Autodesk Inventor part; units mm, degrees
ref_plane "YZ Plane" through (0, 0, 0) normal (1, 0, 0) x (0, 1, 0)
ref_plane "XZ Plane" through (0, 0, 0) normal (0, 1, 0) x (-1, 0, 0)
ref_plane "XY Plane" through (0, 0, 0) normal (0, 0, 1) x (1, 0, 0)
sketch "Sketch6" plane through (0, 0, 0) normal (0, 1, 0) x (-1, 0, 0)
  line L0 (4.5, -6.1) -> (60.5, -6.1)
  line L1 (60.5, -6.1) -> (60.5, -90.9)
  line L2 (4.5, -90.9) -> (4.5, -6.1)
  line L3 (65.1201, -97) -> (0, -97)
  line L4 (0, -97) -> (0, 0)
  line L5 (0, 0) -> (65.1201, 0)
  line L6 (65.1201, 0) -> (65.1201, -97)
  line L7 (60.5, -90.9) -> (4.5, -90.9)
  line L8 (102.5, -48.5) -> (-37.5, -48.5)
  line L9 (32.5, -118.5) -> (32.5, 21.5)
  circle A0 centre (32.5, -48.5) radius 70
  line L10 (102.5, -48.5) -> (67.5, -109.1218)
  line L11 (67.5, -109.1218) -> (-2.5, -109.1218)
  line L12 (-2.5, -109.1218) -> (-37.5, -48.5)
  line L13 (-37.5, -48.5) -> (-2.5, 12.1218)
  line L14 (-2.5, 12.1218) -> (67.5, 12.1218)
  line L15 (67.5, 12.1218) -> (102.5, -48.5)
  line L16 (32.5, 12.1218) -> (85, -18.1891)
  line L17 (85, -18.1891) -> (85, -78.8109)
  line L18 (85, -78.8109) -> (32.5, -109.1218)
  line L19 (32.5, -109.1218) -> (-20, -78.8109)
  line L20 (-20, -78.8109) -> (-20, -18.1891)
  line L21 (-20, -18.1891) -> (32.5, 12.1218)
  line L22 (32.5, 12.1218) -> (47.5, 12.1218)
  line L23 (47.5, 12.1218) -> (47.5, 5.6218)
  line L24 (47.5, 5.6218) -> (17.5, 5.6218)
  line L25 (17.5, 5.6218) -> (17.5, 12.1218)
  line L26 (47.5, 5.6218) -> (56.6924, 5.6218) construction
  line L27 (17.5, 8.8718) -> (20, 8.8718)
  line L28 (47.5, 8.8718) -> (45, 8.8718)
  line L29 (45, 8.8718) -> (45, 10.1218)
  line L30 (45, 10.1218) -> (20, 10.1218)
  line L31 (20, 10.1218) -> (20, 7.6218)
  line L32 (20, 7.6218) -> (45, 7.6218)
  line L33 (45, 7.6218) -> (45, 10.1218)
  line L34 (67.5, 12.1218) -> (32.5, -48.5)
  line L35 (32.5, -48.5) -> (67.5, -109.1218)
  line L36 (47.5, 5.6218) -> (56.6924, 5.6218)
  line L37 (17.5, 5.6218) -> (11, 5.6218)
  line L38 (17.5, 12.1218) -> (11, 5.6218)
  line L39 (17.5, 12.1218) -> (26.6924, 12.1218) construction
  line L40 (47.5, 12.1218) -> (54, 5.6218)
  line L41 (85, -18.1891) -> (77.5, -5.1987)
  line L42 (77.5, -5.1987) -> (71.8708, -8.4487)
  line L43 (71.8708, -8.4487) -> (86.8708, -34.4295)
  line L44 (86.8708, -34.4295) -> (92.5, -31.1795)
  line L45 (71.8708, -8.4487) -> (67.2746, -0.4879) construction
  line L46 (89.6854, -32.8045) -> (88.4354, -30.6394)
  line L47 (74.6854, -6.8237) -> (75.9354, -8.9888)
  line L48 (75.9354, -8.9888) -> (77.0179, -8.3638)
  line L49 (77.0179, -8.3638) -> (89.5179, -30.0144)
  line L50 (89.5179, -30.0144) -> (87.3529, -31.2644)
  line L51 (87.3529, -31.2644) -> (74.8529, -9.6138)
  line L52 (74.8529, -9.6138) -> (77.0179, -8.3638)
  line L53 (71.8708, -8.4487) -> (67.2746, -0.4879)
  line L54 (86.8708, -34.4295) -> (90.1208, -40.0587)
  line L55 (92.5, -31.1795) -> (90.1208, -40.0587)
  line L56 (92.5, -31.1795) -> (87.9038, -23.2187) construction
  line L57 (77.5, -5.1987) -> (68.6208, -2.8196)
  line L58 (71.8708, -88.5513) -> (67.2746, -96.5121) construction
  line L59 (74.6854, -90.1763) -> (75.9354, -88.0112)
  line L60 (74.8529, -87.3862) -> (77.0179, -88.6362)
  line L61 (77.5, -91.8013) -> (71.8708, -88.5513)
  line L62 (77.5, -91.8013) -> (68.6208, -94.1804)
  line L63 (71.8708, -88.5513) -> (67.2746, -96.5121)
  line L64 (77.0179, -88.6362) -> (89.5179, -66.9856)
  line L65 (87.3529, -65.7356) -> (74.8529, -87.3862)
  line L66 (71.8708, -88.5513) -> (86.8708, -62.5705)
  line L67 (89.5179, -66.9856) -> (87.3529, -65.7356)
  line L68 (89.6854, -64.1955) -> (88.4354, -66.3606)
  line L69 (86.8708, -62.5705) -> (92.5, -65.8205)
  line L70 (86.8708, -62.5705) -> (90.1208, -56.9413)
  line L71 (92.5, -65.8205) -> (90.1208, -56.9413)
  line L72 (94.9944, -48.5) -> (63.7472, -102.6218)
  line L73 (63.7472, -102.6218) -> (1.2528, -102.6218)
  line L74 (1.2528, -102.6218) -> (-29.9944, -48.5)
  line L75 (-29.9944, -48.5) -> (1.2528, 5.6218)
  line L76 (1.2528, 5.6218) -> (63.7472, 5.6218)
  line L77 (63.7472, 5.6218) -> (94.9944, -48.5)
  line L78 (74.8529, -87.3862) -> (73.1208, -86.3862)
  line L79 (87.3529, -65.7356) -> (85.6208, -64.7356)
  line L80 (87.3529, -31.2644) -> (85.6208, -32.2644)
  line L81 (74.8529, -9.6138) -> (73.1208, -10.6138)
  line L82 (45, 7.6218) -> (45, 5.6218)
  line L83 (20, 7.6218) -> (20, 5.6218)
  line L84 (60.5, -90.9) -> (4.4985, -90.9)
  line L85 (4.4985, -90.9) -> (4.4985, -97)
  line L86 (4.4985, -97) -> (60.5, -97)
  line L87 (60.5, -97) -> (60.5, -90.9)
  line L88 (60.5, -6.1) -> (4.4985, -6.1)
  line L89 (4.4985, -6.1) -> (4.4985, 0)
  line L90 (4.4985, 0) -> (60.5, 0)
  line L91 (60.5, 0) -> (60.5, -6.1)
  line L92 (-29.9944, -48.5) -> (-22.9944, -48.5)
  line L93 (-29.9944, -48.5) -> (-28.2944, -48.5)
  line L94 (-28.2944, -48.5) -> (-22.9944, -48.5)
  circle A1 centre (-26.9944, -48.5) radius 1.5
  line L95 (-29.9944, -48.5) -> (-23.9944, -48.5)
  line L96 (-23.9944, -48.5) -> (-26.9944, -53.6962)
  line L97 (-23.9944, -48.5) -> (-26.9944, -43.3038)
  point P0 (-27.5473, -52.7386)
  point P1 (-28.2775, -45.5261)
  dimension "d44" = 97
  dimension "d77" = 140
  dimension "d87" = 15
  dimension "d88" = 6.5
  dimension "d89" = 30
  dimension "d91" = 2.5
  dimension "d92" = 2.5
  dimension "d95" = 1.25
  dimension "d96" = 25
  dimension "d97" = 2.5
  dimension "d98" = 25
  dimension "d99" = 135
  dimension "d100" = 0
  dimension "d114" = 1.7
  dimension "d117" = 3
  dimension "d121" = 3
  dimension "d123" = 6
extrude "Fronte" add sketch "Sketch6" along normal blind 2.5 contours L89 L21 L5 L9 L0 | L2 L8 L4 L21 L89 | L9 L5 L16 L34 L0 | L2 L85 L19 L4 L8 | L89 L5 L21 | L21 L4 L5 L89 | L34 L16 L91 L0 | L9 L24 L16 L5 | L5 L21 L24 L9 | L7 L9 L3 L19 L85 | L8 L20 L75 L21 L4 | L4 L19 L74 L20 L8 | L21 L75 L76 L37 L24 L5 L4 | L91 L16 L6 L8 L1 | L34 L91 L16 | L16 L5 L34 | L8 L6 L18 L87 L1 | L7 L35 L18 L3 L9 | L7 L87 L18 L35 | L16 L24 L36 L76 L34 L5 | L24 L21 L32 L9 | L9 L32 L16 L24 | L85 L3 L4 L19 | L19 L3 L85 | L4 L3 L19 L73 L74 | L20 L74 L96 L8 | L8 L97 L75 L20 | L75 L20 L21 | L21 L13 L14 L38 L76 L75 | L24 L83 L32 L21 | L91 L5 L6 L16 | L34 L77 L53 L43 L16 L6 L5 | L8 L17 L66 L18 L6 | L6 L16 L43 L17 L8 | L9 L73 L19 L3 | L3 L18 L73 L9 | L35 L3 L18 | L18 L87 L35 | L16 L32 L82 L24 | L32 L21 L30 L9 | L9 L30 L16 L32 | L74 L73 L19 L11 L12 | L19 L20 L74 | L20 L12 L8 L74 | L75 L8 L13 L20 | L32 L31 L30 L21 | L24 L25 L27 L31 L83 | L76 L36 L40 L14 L34 | L34 L15 L57 L53 L77 | L18 L6 L3 L87 | L18 L66 L63 L72 L35 L3 L6 | L17 L43 L54 L77 L8 | L8 L72 L70 L66 L17 | L3 L35 L73 L18 | L73 L18 L9 | L9 L19 L73 | L16 L30 L29 L33 L32 | L82 L33 L28 L23 L24 | L30 L21 L9 | L9 L16 L30 | L96 L74 L8 A1 | L8 A1 L75 L97 | L38 L25 L37 | L30 L31 L27 L25 L14 L21 | L43 L81 L51 L16 | L16 L51 L17 L43 | L66 L17 L65 L18 | L18 L65 L78 L66 | L77 L55 L15 L8 | L8 L10 L71 L72 | L17 L51 L80 L43 | L66 L79 L65 L17 | L73 L35 L11 L18 | L72 L63 L62 L10 L35 | L16 L14 L23 L28 L29 L30 | L23 L40 L36 | A1 L8 | L8 A1 | L51 L52 L48 L49 L16 | L16 L49 L17 L51 | L43 L42 L47 L52 L81 | L15 L16 L49 L48 L47 L42 | L42 L53 L57 | L65 L17 L64 L18 | L18 L64 L60 L65 | L78 L60 L59 L61 L66 | L71 L69 L70 | L54 L44 L55 | L17 L49 L50 L51 | L80 L50 L46 L44 L43 | L65 L67 L64 L17 | L66 L69 L68 L67 L79 | L16 L17 L49 | L10 L17 L64 L67 L68 L69 | L44 L46 L50 L49 L17 L15 | L64 L17 L18 | L18 L10 L61 L59 L60 L64 | L61 L62 L63
properties part number "FrontalinoWood" material "Wood (Walnut)"
The model under review builds one solid part; all positions refer to its coordinate system, in mm. Round coordinates to 2 decimals unless told otherwise and drop trailing zeros. Order: outer loops, then holes, each group sorted by start corner. A loop starts at its lowest first (then second) coordinate and runs counter-clockwise, first axis right, second up. Notation, with made-up numbers: (-22, 78.25) -> (27, 78.25) arc R30 cw to (27, 100.25) -> close; hole circle Ø4 at (63.5, 16). An arc over 180 degrees is marked (long way). One line per item, written item: value. Start each with the question number.
Q1. Take a section at D-D (z = -2). Write out the cut boundary in (x, y).
Q2. Take a section at A-A (x = -39). Write out the cut boundary in (y, z), and give its area (3 significant figures).
Q3. Take a section at C-C (y = 1.3). Write out the cut boundary in (x, z).
Q4. Take a section at B-B (z = -88.5). Write out the cut boundary in (x, y).
Q5. Wall thickness on line 1 (Z direction, x = -47, y = 0.1); line 2 (X direction, y = 2, z = -55.5); line 3 (X direction, y = 2, z = -14): over which ranges is each line inside the solid? List them lowest first.
Q6. Clearance check with a flat-ended pin moving along its axis: pin 1 Ø1.2 at (y, z) = (1, -50.5) entering from +X. State where the tip first meets the part, or that it passes through.
Reported:
1. outline: (-75.65, 0) -> (10.65, 0) -> (10.65, 2.5) -> (-75.65, 2.5) -> close
2. outline: (0, -109.12) -> (2.5, -109.12) -> (2.5, -90.9) -> (0, -90.9) -> close; (0, -6.1) -> (2.5, -6.1) -> (2.5, 12.12) -> (0, 12.12) -> close
2. area: 91.1 mm2
3. outline: (-102.5, -48.5) -> (-67.5, -109.12) -> (2.5, -109.12) -> (37.5, -48.5) -> (2.5, 12.12) -> (-67.5, 12.12) -> close; hole (-60.5, -90.9) -> (-4.5, -90.9) -> (-4.5, -6.1) -> (-60.5, -6.1) -> close
4. outline: (-79.41, 0) -> (-60.5, 0) -> (-60.5, 2.5) -> (-79.41, 2.5) -> close; (-4.5, 0) -> (14.41, 0) -> (14.41, 2.5) -> (-4.5, 2.5) -> close
5. line 1: z = -109.12 to -90.9, -6.1 to 12.12
5. line 2: x = -98.46 to -60.5, -4.5 to 33.46
5. line 3: x = -82.58 to -60.5, -4.5 to 17.58
6. pin 1: stops at x = 36.69
